Here's how the part is built. I have some questions about the finished solid (model axes, mm). Face numbers are marked on the shaded views. A direction names the side the tool comes from. Coordinates: 2 decimals unless noted, no trailing zeros. Order: outer loops, then holes, each group sorted by start corner. A loop starts at its lowest first (then second) coordinate and runs counter-clockwise, first axis right, second up. Notation, with made-up numbers: (21.5, 38) - (68.5, 38) arc R19 ccw to (68.5, 61) - close; hole circle Ø10 at (33, 43). An arc over 180 degrees is marked (long way). Use one line per item in the form item = value. Start each with the question number.
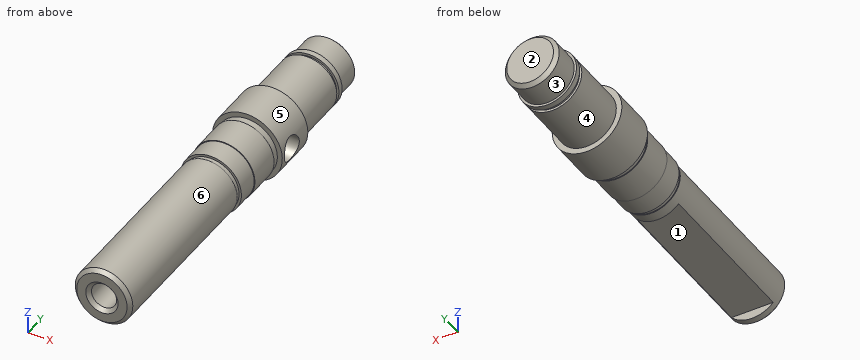
from build123d import *

# Parameters (mm, degrees)
ENL_V_START             = -5.5
ESQUISSE2_W             = 11.618950038
ESQUISSE2_H             = 44.4
ENL_V_MAT_EXTRU_1_DEPTH = 103.375761874
ENL_V_MAT_EXTRU_2_DEPTH = 108.875761874
ESQUISSE6_R             = 3.5
ENL_V_MAT_EXTRU_3_DEPTH = 78
CHANFREIN1_SIZE         = 1


with BuildPart() as part:
    # Esquisse1 → Révolution1 (revolve)
    with BuildSketch(Plane.XY, mode=Mode.PRIVATE) as r_volution1_sk:
        Polygon((0, 0), (-7, 0), (-8, 1), (-8, 50), (-7.75, 50), (-7.75, 51.3), (-8.4, 51.3), (-8.4, 57.3), (-8.6, 57.3), (-8.6, 66.3), (-8.33, 66.3), (-8.33, 68.3), (-9.7, 68.3), (-9.7, 80.3), (-8.15, 80.3), (-8.15, 96.5), (-7.5, 96.5), (-7.5, 97.5), (-8.15, 97.5), (-8.15, 99), (-7.5, 99), (-7.5, 106), (-6.5, 107), (0, 107), align=None)
    revolve(r_volution1_sk.sketch.rotate(Axis((0, 107, 0), (0, -1, 0)), 270), axis=Axis((0, 107, 0), (0, -1, 0)))

    # Esquisse2 → Enlèv. mat.-Extru.1 (cut, through all)
    with BuildSketch(Plane.XY.offset(ENL_V_START)):
        with Locations((0, 24.9)):
            Rectangle(ESQUISSE2_W, ESQUISSE2_H)
    extrude(amount=-ENL_V_MAT_EXTRU_1_DEPTH, mode=Mode.SUBTRACT)

    # Esquisse5 → Enlèv. mat.-Extru.2 (cut, through all)
    with BuildSketch(Plane(origin=(0, 0, 0), x_dir=(0, 0, -1), z_dir=(1, 0, 0))):
        with BuildLine():
            ThreePointArc((0, 76.3), (-3.5, 72.8), (0, 69.3))
            ThreePointArc((0, 69.3), (3.5, 72.8), (0, 76.3))
        make_face()
    extrude(amount=ENL_V_MAT_EXTRU_2_DEPTH, mode=Mode.SUBTRACT)

    # Esquisse6 → Enlèv. mat.-Extru.3 (cut)
    with BuildSketch(Plane.XZ):
        with Locations(Location((0, 0, 0), (0, 0, 270))):
            Circle(ESQUISSE6_R)
    extrude(amount=-ENL_V_MAT_EXTRU_3_DEPTH, mode=Mode.SUBTRACT)

    # Chanfrein1
    chanfrein1_edges = [part.edges().sort_by_distance(p)[0] for p in [
        (0, 0, 3.5),
    ]]
    chamfer(chanfrein1_edges, length=CHANFREIN1_SIZE)


solid = part.part
1) Suppose I cut it at A-A, the plane y = 11. List the corners of the cut face in (x, z) for me.
2) If we mould it in two halves opening along Y, with no side actions, what happens to the marked faces 1, 2 and 3? For each: pulls with the +Y half, pulls with the -Y half, needs draft (parallel to the pull), parting line crosses it, or undercut.
3) For pin 1 (3.5 mm diameter, centred on x = 1.5, z = 1.5, fed in from -Y); pin 2 (1 mm diameter, centred on x = -6.5, z = 7.5, fed in from -Y); pin 3 (8 mm diameter, centred on x = 0, z = 0, fed in from -Y), each with a flat end and sliding along its axis, tell me the tip position at first contact or that it passes through.
4) Suppose I cut it at B-B, the plane y = 72.8. List the corners of the cut face in (x, z) for me.
5) I need wall thicknesses on probe 1 along Y at (x, z) = (5.25, 0); probe 2 along Y at (x, z) = (-4.75, 7); probe 3 along Y at (x, z) = (-8.5, 3.25). Which ranges of each line are inside material? Lowest first, please. Write a range as [from, to].
6) Which directions (+Z, -Z, +X, -X, +Y, -Y) give clear straight access to the entire face, cutting with the end or side of a thin tool? Please do the marked faces 4, 5 and 6.
From the geometry:
q1.outline = (-5.81, -5.5) - (5.81, -5.5) arc R8 ccw (long way) to start; hole circle Ø7 at (0, 0)
q2.face_1 = undercut
q2.face_2 = pulls with the +Y half
q2.face_3 = needs draft
q3.pin_1 = 0.63
q3.pin_2 = 68.3
q3.pin_3 = 0.5
q4.outline = (0, -3.5) arc R3.5 cw to (0, 3.5) - (9.05, 3.5) arc R9.7 ccw (long way) to (9.05, -3.5) - close
q5.probe_1 = [0, 69.3], [76.3, 107]
q5.probe_2 = [57.3, 66.3], [68.3, 80.3]
q5.probe_3 = [68.3, 80.3]
q6.face_4 = +Y
q6.face_5 = +Y, -Y
q6.face_6 = -Y
